```python
from build123d import *

# Parameters (mm, degrees)
SKETCH1_W           = 700
SKETCH1_H           = 588
BOSS_EXTRUDE1_DEPTH = 6
FILLET1_R           = 20
SKETCH2_R           = 14.4
SKETCH2_W           = 71.3
SKETCH2_H           = 24.4
CUT_EXTRUDE1_DEPTH  = 10


with BuildPart() as part:
    # Sketch1 → Boss-Extrude1 (new body)
    with BuildSketch(Plane.XY):
        Rectangle(SKETCH1_W, SKETCH1_H)
    extrude(amount=BOSS_EXTRUDE1_DEPTH)

    # Fillet1
    fillet1_edges = [part.edges().sort_by_distance(p)[0] for p in [
        (350, -294, 3),
        (-350, -294, 3),
        (-350, 294, 3),
        (350, 294, 3),
    ]]
    fillet(fillet1_edges, radius=FILLET1_R)

    # Sketch2 → Cut-Extrude1 (cut)
    with BuildSketch(Plane.XY.offset(6)):
        with Locations((-315, -225)):
            Circle(SKETCH2_R)
        with Locations((-279.35, -266.8)):
            Rectangle(SKETCH2_W, SKETCH2_H)
        with BuildLine():
            Line((-262, -225), (302, -225))
            ThreePointArc((302, -225), (309.071067812, -222.071067812), (312, -215))
            Line((312, -215), (312, 215))
            ThreePointArc((312, 215), (309.071067812, 222.071067812), (302, 225))
            Line((302, 225), (-262, 225))
            ThreePointArc((-262, 225), (-269.071067812, 222.071067812), (-272, 215))
            Line((-272, 215), (-272, -215))
            ThreePointArc((-272, -215), (-269.071067812, -222.071067812), (-262, -225))
        make_face()
    extrude(amount=-CUT_EXTRUDE1_DEPTH, mode=Mode.SUBTRACT)


solid = part.part
```
The listing builds one solid part. Answer for the finished solid, in the listing's coordinates (mm). Coordinates: 2 decimals unless noted, no trailing zeros. Write each loop counter-clockwise with the first axis right and the second up, starting at its lowest first coordinate (ties: lowest second). Pieces come first, ordered by that corner, then holes.
Q1. The mould has two halves that part along Y. Classify faces 1 (the cylindrical face through (-307.259, -212.858, 3.042)), 2 (the flat face through (-79, 241, 0)), 3 (the cylindrical face through (-344.297, 287.986, 3.042)): released by +Y, released by -Y, zero draft, split by the parting line, or undercut.
Returned:
face 1: undercut
face 2: zero draft
face 3: released by +Y
Q2. Section A-A, the plane x = -79.5 is taken. Write down the section's boundary in (y, z), then the cut area to 3 significant figures.
Returned:
outline: (-294, 0) - (-225, 0) - (-225, 6) - (-294, 6) - close; (225, 0) - (294, 0) - (294, 6) - (225, 6) - close
area: 828 mm2
Q3. Section C-C, the plane y = -176.5 is taken. Write down the section's boundary in (x, z).
Returned:
outline: (-350, 0) - (-272, 0) - (-272, 6) - (-350, 6) - close; (312, 0) - (350, 0) - (350, 6) - (312, 6) - close
Q4. Section B-B, the plane z = 0.9 is taken. Write down the section's boundary in (x, y), then the cut area to 3 significant figures.
Returned:
outline: (-350, -274) arc R20 ccw to (-330, -294) - (330, -294) arc R20 ccw to (350, -274) - (350, 274) arc R20 ccw to (330, 294) - (-330, 294) arc R20 ccw to (-350, 274) - close; hole circle Ø28.8 at (-315, -225); hole (-315, -279) - (-243.7, -279) - (-243.7, -254.6) - (-315, -254.6) - close; hole (-272, -215) arc R10 ccw to (-262, -225) - (302, -225) arc R10 ccw to (312, -215) - (312, 215) arc R10 ccw to (302, 225) - (-262, 225) arc R10 ccw to (-272, 215) - close
area: 146,000 mm2
Q5. Find the intervals of material crossed by line 1 along Y through (x, z) = (168, 3.75); line 2 along X through (y, z) = (-71, 5.7); line 3 along Y through (x, z) = (-299, 2.95), in increasing order.
Returned:
line 1: y = -294 to -225, 225 to 294
line 2: x = -350 to -272, 312 to 350
line 3: y = -294 to -279, -254.6 to 294
